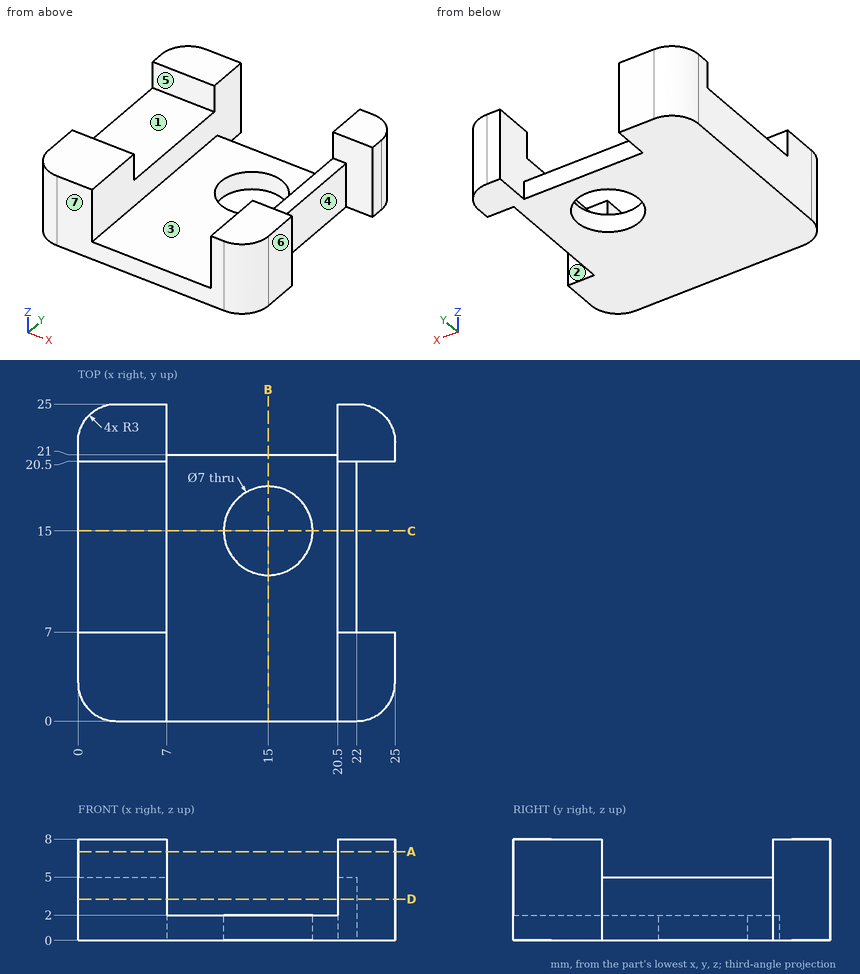
Source: three-view drawing plus pictorial views. Frame: mm from the lowest corner of the part. A direction names the side the tool comes from. Coordinates: 2 decimals unless noted, no trailing zeros. Order: outer loops, then holes, each group sorted by start corner. A loop starts at its lowest first (then second) coordinate and runs counter-clockwise, first axis right, second up. Notation, with made-up numbers: M 64.5,61 L 85.5,61 A22 cw 85.5,89 Z; hole C -12,-34.5 d6. An arc over 180 degrees is marked long. One line per question, with ' | ' between items. Start each with the question number.
Item 1: Cut plane B-B, the plane x = 15. Return the cut outline in (y, z), then the cut area to 3 significant figures.
Item 2: Cut plane A-A, the plane z = 7. Return the cut outline in (x, y), then the cut area to 3 significant figures.
Item 3: Ray query, probe 1 along X at (y, z) = (15, 0.8); probe 2 along X at (y, z) = (21.75, 4); probe 3 along Y at (x, z) = (15, 1.45). Return the intervals inside material, ascending. Write a range as [from, to].
Item 4: Set-up query: the marked faces 1, 2, 3 and 4. Return all of +Z, -Z, +X, -X, +Y, -Y with unobstructed straight access to the full face (end or side cutting, diameter ignored); none if empty.
Item 5: Pin query (flat end, axial travel): pin 1 Ø1.5 at (y, z) = (13.5, 2) entering from +X; pin 2 Ø0.8 at (x, y) = (21, 13) entering from +Z; pin 3 Ø1.5 at (x, z) = (2, 6) entering from -Y. Return the tip coordinate at first contact, or that it passes through.
Item 6: Cut plane C-C, the plane y = 15. Return the cut outline in (x, z), then the cut area to 3 significant figures.
Item 7: Cut plane D-D, the plane z = 3.25. Return the cut outline in (x, y), then the cut area to 3 significant figures.
Item 8: Draft query along Y for the marked faces 5, 6 and 7. Return one class per face: released by +Y, released by -Y, zero draft, split by the parting line, or undercut.
A:
1) outline: M 0,0 L 11.5,0 L 11.5,2 L 0,2 Z; M 18.5,0 L 21,0 L 21,2 L 18.5,2 Z | area: 28.0 mm2
2) outline: M 0,3 A3 ccw 3,0 L 7,0 L 7,7 L 0,7 Z; M 0,20.5 L 7,20.5 L 7,25 L 3,25 A3 ccw 0,22 Z; M 20.5,0 L 22,0 A3 ccw 25,3 L 25,7 L 20.5,7 Z; M 20.5,20.5 L 25,20.5 L 25,22 A3 ccw 22,25 L 20.5,25 Z | area: 125 mm2
3) probe 1: x = [0, 11.5], [18.5, 22] | probe 2: x = [0, 7], [20.5, 25] | probe 3: y = [0, 11.5], [18.5, 21]
4) face 1: +Z, +X, -X | face 2: +Z, +X | face 3: +Z, +Y, -Y | face 4: +Z, -Z, +X
5) pin 1: stops at x = 22 | pin 2: stops at z = 5 | pin 3: stops at y = 0.01
6) outline: M 0,0 L 11.5,0 L 11.5,2 L 7,2 L 7,5 L 0,5 Z; M 18.5,0 L 22,0 L 22,5 L 20.5,5 L 20.5,2 L 18.5,2 Z | area: 55.5 mm2
7) outline: M 0,3 A3 ccw 3,0 L 7,0 L 7,25 L 3,25 A3 ccw 0,22 Z; M 20.5,0 L 22,0 A3 ccw 25,3 L 25,7 L 22,7 L 22,20.5 L 25,20.5 L 25,22 A3 ccw 22,25 L 20.5,25 Z | area: 239 mm2
8) face 5: undercut | face 6: zero draft | face 7: released by -Y
